Model file for the job. Use its own axes, mm. Face numbers are marked on the shaded views. A direction names the side the tool comes from. Round coordinates to 2 decimals unless told otherwise and drop trailing zeros. Order: outer loops, then holes, each group sorted by start corner. A loop starts at its lowest first (then second) coordinate and runs counter-clockwise, first axis right, second up. Notation, with made-up numbers: (44, 25.5) -> (85, 25.5) arc R8 cw to (85, 31.5) -> close; hole circle Ø8 at (52.25, 16). An arc over 180 degrees is marked (long way). Use CSV: the item, a comma, the result in double quotes.
```python
from build123d import *

# Parameters (mm, degrees)
EXTRUDE_1_DEPTH     = 10
SKETCH_2_R          = 1.646034056
CUT_EXTRUDE_1_DEPTH = 84.366660003


with BuildPart() as part:
    # 草图1 → 凸台-拉伸1 (new body)
    with BuildSketch(Plane(origin=(0, 0, 0), x_dir=(1, 0, 0), z_dir=(0, 1, 0))):
        Polygon((-8.112254188, -35), (-8.112254188, -75), (6.887745812, -75), (6.887745812, -35), (35, -35), (35, 35), (-35, 35), (-35, -35), align=None)
        with BuildLine():
            Line((-20, 25), (20, 25))
            ThreePointArc((20, 25), (23.535533906, 23.535533906), (25, 20))
            Line((25, 20), (25, -20))
            ThreePointArc((25, -20), (23.535533906, -23.535533906), (20, -25))
            Line((20, -25), (-20, -25))
            ThreePointArc((-20, -25), (-23.535533906, -23.535533906), (-25, -20))
            Line((-25, -20), (-25, 20))
            ThreePointArc((-25, 20), (-23.535533906, 23.535533906), (-20, 25))
        make_face(mode=Mode.SUBTRACT)
    extrude(amount=EXTRUDE_1_DEPTH)

    # 草图2 → 切除-拉伸1 (cut, through all)
    with BuildSketch(Plane(origin=(0, 10, 0), x_dir=(1, 0, 0), z_dir=(0, 1, 0))):
        with Locations(Location((0, -71.838140911, 0), (0, 0, 270))):
            Circle(SKETCH_2_R)
    extrude(amount=-CUT_EXTRUDE_1_DEPTH, mode=Mode.SUBTRACT)


solid = part.part
```
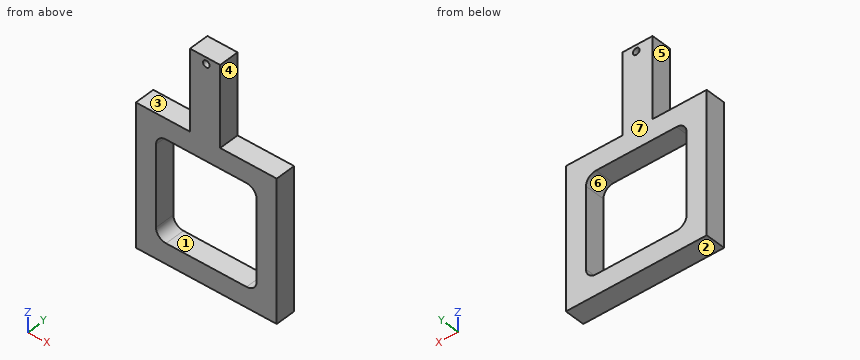
Q1. Cut at C-C (z = -6.5). Give the cut face in (x, y).
From the geometry:
outline,"(-35, 0) -> (-25, 0) -> (-25, 10) -> (-35, 10) -> close; (25, 0) -> (35, 0) -> (35, 10) -> (25, 10) -> close"
Q2. Probe line 1 along Z through (x, y) = (18, 2); line 2 along Z through (x, y) = (-8, 7.25). List the from-to ranges inside material, lowest first.
From the geometry:
line 1,"z = -35 to -25, 25 to 35"
line 2,"z = -35 to -25, 25 to 75"
Q3. Cut at D-D (x = 0). Give the cut face in (y, z).
From the geometry:
outline,"(0, -35) -> (10, -35) -> (10, -25) -> (0, -25) -> close; (0, 25) -> (10, 25) -> (10, 70.19) -> (0, 70.19) -> close; (0, 73.48) -> (10, 73.48) -> (10, 75) -> (0, 75) -> close"
Q4. Which spindle directions (+Z, -Z, +X, -X, +Y, -Y) get a long thin tool onto all of the face, cutting with end or side? Do the marked faces 1, 2, 3 and 4. Say none if no direction does.
From the geometry:
face 1,"+Y, -Y"
face 2,"-Z, +X, -X, +Y, -Y"
face 3,"+Z, -X, +Y, -Y"
face 4,"+Z, +X, +Y, -Y"
Q5. Cut at A-A (x = -7). Give the cut face in (y, z).
From the geometry:
outline,"(0, -35) -> (10, -35) -> (10, -25) -> (0, -25) -> close; (0, 25) -> (10, 25) -> (10, 75) -> (0, 75) -> close"
Q6. Cut at B-B (y = 5.5). Give the cut face in (x, z), plus the area to 3 significant figures.
From the geometry:
outline,"(-35, -35) -> (35, -35) -> (35, 35) -> (6.89, 35) -> (6.89, 75) -> (-8.11, 75) -> (-8.11, 35) -> (-35, 35) -> close; hole (-25, -20) arc R5 ccw to (-20, -25) -> (20, -25) arc R5 ccw to (25, -20) -> (25, 20) arc R5 ccw to (20, 25) -> (-20, 25) arc R5 ccw to (-25, 20) -> close; hole circle Ø3.29 at (0, 71.84)"
area,"3,010 mm²"
Q7. Pin check, flat tips, straight feed: pin 1 (5 mm diameter, centred on y = 7, z = 61, fed in from +X); pin 2 (5 mm diameter, centred on y = 6, z = 59.5, fed in from -X); pin 3 (5 mm diameter, centred on x = -26.5, y = 7, fed in from +Z). Stop position of each tip, or through.
From the geometry:
pin 1,"stops at x = 6.89"
pin 2,"stops at x = -8.11"
pin 3,"stops at z = 35"
Q8. Mould opens along X. For the marked faces 5, 6 and 7 say: +X half, -X half, draft (parallel to the pull), parting line (faces both ways), or undercut.
From the geometry:
face 5,"-X half"
face 6,"undercut"
face 7,"draft"
